CAD build for the part. Positions are in the model's coordinates, mm. Give positions to 0.01 mm unless a question says otherwise; leave off trailing zeros. Loops run counter-clockwise (first coordinate to the right, second up) from the corner with the lowest first, then second, coordinate; pieces in that order, holes last.
Item 1: Probe probe 1 along X at (y, z) = (1.7, 45); probe 2 along Z at (x, y) = (125, 1.15). List the from-to ranges inside material, lowest first.
Item 2: Drop flat-ended pins along their axis: P1, Ø1, axis at y = 1, z = -51.5, coming from the +X side; P2, Ø0.6, axis at y = 1, z = -50.5, coming from the -X side; P3, Ø0.6, axis at x = 127.5, y = 0.5, coming from the -Z side. Give the stop position or say it passes through.
Item 3: Saw through at B-B on x = 236.5. Give the cut face in (y, z).
from build123d import *

# Parameters (mm, degrees)
SKETCH_1_W      = 40
SKETCH_1_H      = 2
SKETCH_1_W_2    = 50
SKETCH_1_W_3    = 350
SKETCH_1_H_2    = 100
EXTRUDE_1_DEPTH = 2
SKETCH_2_W      = 2
SKETCH_2_H      = 40
EXTRUDE_2_DEPTH = 2


with BuildPart() as part:
    # 草图1 → 凸台-拉伸1 (new body)
    with BuildSketch(Plane(origin=(0, 0, 0), x_dir=(1, 0, 0), z_dir=(0, 1, 0))):
        with Locations((60, 51)):
            Rectangle(SKETCH_1_W, SKETCH_1_H)
        with Locations((60, -51)):
            Rectangle(SKETCH_1_W, SKETCH_1_H)
        with Locations((175, 51)):
            Rectangle(SKETCH_1_W_2, SKETCH_1_H)
        with Locations((175, -51)):
            Rectangle(SKETCH_1_W_2, SKETCH_1_H)
        with Locations((295, 51)):
            Rectangle(SKETCH_1_W_2, SKETCH_1_H)
        with Locations((295, -51)):
            Rectangle(SKETCH_1_W_2, SKETCH_1_H)
        with Locations((175, 0)):
            Rectangle(SKETCH_1_W_3, SKETCH_1_H_2)
    extrude(amount=EXTRUDE_1_DEPTH)

    # 草图2 → 凸台-拉伸2 (add)
    with BuildSketch(Plane(origin=(0, 0, 0), x_dir=(1, 0, 0), z_dir=(0, 1, 0))):
        with Locations((351, 0)):
            Rectangle(SKETCH_2_W, SKETCH_2_H)
    extrude(amount=EXTRUDE_2_DEPTH)


solid = part.part
Results below:
1. probe 1: x = 0 to 350
1. probe 2: z = -50 to 50
2. P1: stops at x = 320
2. P2: stops at x = 40
2. P3: stops at z = -50
3. outline: (0, -50) - (2, -50) - (2, 50) - (0, 50) - close
